from build123d import *

# Parameters (mm, degrees)
F3_D            = 3.3
F3_CBORE_D      = 6.5
F3_CBORE_DEPTH  = 3
F3_COPIES_COUNT = 3


# Not quite as in the source:
# - a pattern or mirror of a feature is missing from the dataset's text; its kind, count and spacing are read off the source's solid


with BuildPart() as f1:
    # F0 (on Front) → F1 (revolve)
    with BuildSketch(Plane.XZ):
        Polygon((-8, 4.5), (6, 4.5), (6, 17), (0, 17), (0, 25.5), (-2.5, 25.5), (-2.5, 23.875), (-12.5, 23.875), (-12.5, 25.5), (-15, 25.5), (-15, 11), (-8, 11), align=None)
    revolve(axis=Axis((0.8759173031, 0, 0), (1, 0, 0)))

    # F3 (through all)
    with Locations(Plane(origin=(-15, 0, 0), x_dir=(0, -1, 0), z_dir=(-1, 0, 0))):
        with Locations((0, 20)):
            f3 = CounterBoreHole(F3_D / 2, F3_CBORE_D / 2, F3_CBORE_DEPTH)

    # F3_copies: F3 ×3 about axis
    f3_copies_axis = Axis((0, 0, 0), (1, 0, 0))
    for i in range(1, F3_COPIES_COUNT):
        add(f3.rotate(f3_copies_axis, i * 360 / F3_COPIES_COUNT), mode=Mode.SUBTRACT)


solid = f1.part
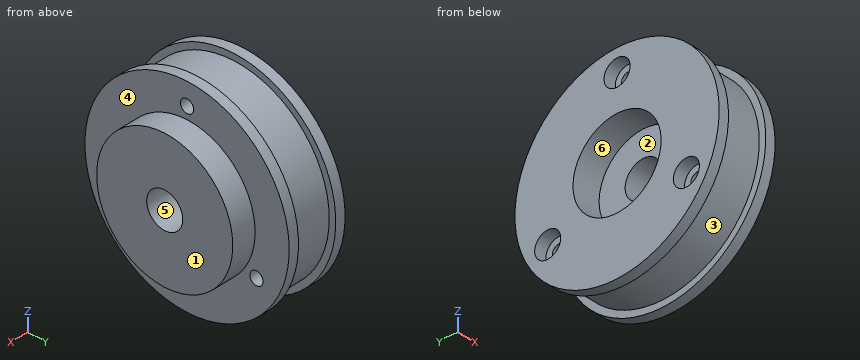
Design review of the part built by this model. Coordinates are the model's own, in mm. Face numbers are marked on the shaded views. A direction names the side the tool comes from. Give positions to 0.01 mm unless a question says otherwise; leave off trailing zeros. Write each loop counter-clockwise with the first axis right and the second up, starting at its lowest first coordinate (ties: lowest second). Pieces come first, ordered by that corner, then holes. Notation, with made-up numbers: M 59,28 L 118,28 A28 cw 118,50 Z; hole C 23.25,57 d8. An arc over 180 degrees is marked long. Return JSON: item names as keys, results as strings. Group by question number.
Item 1: Wall thickness on line 1 along Z through (x, y) = (-5.25, 0) (3 decimals); line 2 along Z through (x, y) = (-13.9, 0); line 3 along Y through (x, z) = (-4, 0) (3 decimals): over which ranges is each line inside the solid? List them lowest first.
Item 2: Take a section at A-A (y = 0). Count the separate pieces of the cut face and the enclosed holes in it, plus the area to 3 significant figures.
Item 3: Take a section at D-D (z = 20). Give the boundary of the cut face in (x, y).
Item 4: Take a section at B-B (z = 0). Give the boundary of the cut face in (x, y) (3 decimals), plus the area to 4 significant figures.
Item 5: Clearance check with flat-ended pins moving along their axes: pin 1 Ø17.5 at (y, z) = (3.5, -2.5) entering from -X; pin 2 Ø10 at (y, z) = (3, 0) entering from -X; pin 3 Ø6 at (x, z) = (-2.5, 5) entering from -Y; pin 4 Ø1 at (x, z) = (-6.5, -9.5) entering from -Y. State where each tip first meets the part, or that it passes through.
Item 6: Tool access review of the marked faces 4, 5 and 6: name each direction out of +Z, -Z, +X, -X, +Y, -Y from which nothing blocks a thin tool from reaching the whole face with its end or side.
Item 7: The part is to be moulded in two halves that separate along Z. For the marked faces 1, 2 and 3, say which applies: pulls with the +Z half, pulls with the -Z half, needs draft (parallel to the pull), parting line crosses it, or undercut.
Return value:
{
 "1": {"line 1": "z = -23.875 to -4.5, 4.5 to 18.35, 21.65 to 23.875", "line 2": "z = -25.5 to -11, 11 to 16.75, 23.25 to 25.5", "line 3": "y = -23.875 to -4.5, 4.5 to 23.875"},
 "2": {"separate pieces": "3", "enclosed holes": "0", "area": "597 mm2"},
 "3": {"outline": "M -15,-15.82 L -12.5,-15.82 L -12.5,-13.04 L -2.5,-13.04 L -2.5,-15.82 L 0,-15.82 L 0,-1.65 L -12,-1.65 L -12,-3.25 L -15,-3.25 Z; M -15,3.25 L -12,3.25 L -12,1.65 L 0,1.65 L 0,15.82 L -2.5,15.82 L -2.5,13.04 L -12.5,13.04 L -12.5,15.82 L -15,15.82 Z"},
 "4": {"outline": "M -15,-25.5 L -12.5,-25.5 L -12.5,-23.875 L -2.5,-23.875 L -2.5,-25.5 L 0,-25.5 L 0,-17 L 6,-17 L 6,-4.5 L -8,-4.5 L -8,-11 L -15,-11 Z; M -15,11 L -8,11 L -8,4.5 L 6,4.5 L 6,17 L 0,17 L 0,25.5 L -2.5,25.5 L -2.5,23.875 L -12.5,23.875 L -12.5,25.5 L -15,25.5 Z", "area": "656.5 mm2"},
 "5": {"pin 1": "stops at x = -15", "pin 2": "stops at x = -8", "pin 3": "stops at y = -25.42", "pin 4": "stops at y = -22.11"},
 "6": {"face 4": "+X", "face 5": "+X, -X", "face 6": "-X"},
 "7": {"face 1": "needs draft", "face 2": "undercut", "face 3": "parting line crosses it"}
}
